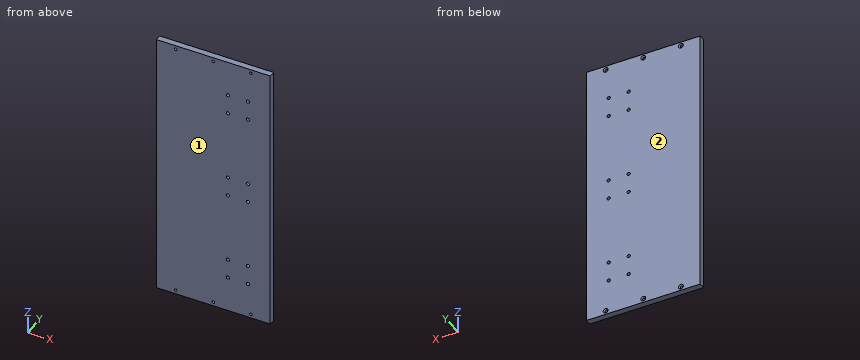
from build123d import *

# Parameters (mm, degrees)
SKETCH1_W                                    = 148
SKETCH1_H                                    = 344
BOSS_EXTRUDE1_DEPTH                          = 8
CSK_FOR_M3_COUNTERSUNK_FLAT_HEAD1_AT_2_COUNT = 2
CSK_FOR_M3_COUNTERSUNK_FLAT_HEAD1_AT_2_PITCH = 49
CSK_FOR_M3_COUNTERSUNK_FLAT_HEAD1_AT_3_COUNT = 2
CSK_FOR_M3_COUNTERSUNK_FLAT_HEAD1_AT_3_PITCH = 98
M5X0_8_TAPPED_HOLE1_D                        = 4.2
LPATTERN1_COUNT                              = 2
LPATTERN1_PITCH                              = 114
LPATTERN1_COL_COUNT                          = 2
LPATTERN1_COL_PITCH                          = 114


with BuildPart() as part:
    # Sketch1 → Boss-Extrude1 (new body)
    with BuildSketch(Plane(origin=(0, 0, 0), x_dir=(1, 0, 0), z_dir=(0, 1, 0))):
        Rectangle(SKETCH1_W, SKETCH1_H)
    extrude(amount=BOSS_EXTRUDE1_DEPTH)

    # Sketch3 → CSK for M3 Countersunk Flat Head1 (revolve, cut)
    with BuildSketch(Plane(origin=(-49, 8, 167), x_dir=(0, 0, 1), z_dir=(1, 0, 0))):
        Polygon((0, 0), (0, 16.021463052), (1.7, 15), (1.7, 1.45), (3.15, 0), align=None)
    csk_for_m3_countersunk_flat_head1 = revolve(axis=Axis((-49, 14.35, 167), (0, -1, 0)), mode=Mode.SUBTRACT)

    # CSK for M3 Countersunk Flat Head1 at 2: CSK for M3 Countersunk Flat Head1 ×2
    with Locations(*[(i * CSK_FOR_M3_COUNTERSUNK_FLAT_HEAD1_AT_2_PITCH, 0, 0) for i in range(1, CSK_FOR_M3_COUNTERSUNK_FLAT_HEAD1_AT_2_COUNT)]):
        add(csk_for_m3_countersunk_flat_head1, mode=Mode.SUBTRACT)

    # CSK for M3 Countersunk Flat Head1 at 3: CSK for M3 Countersunk Flat Head1 ×2
    with Locations(*[(i * CSK_FOR_M3_COUNTERSUNK_FLAT_HEAD1_AT_3_PITCH, 0, 0) for i in range(1, CSK_FOR_M3_COUNTERSUNK_FLAT_HEAD1_AT_3_COUNT)]):
        add(csk_for_m3_countersunk_flat_head1, mode=Mode.SUBTRACT)

    # Mirror1: CSK for M3 Countersunk Flat Head1 across plane
    add(csk_for_m3_countersunk_flat_head1.mirror(Plane.XY), mode=Mode.SUBTRACT)

    # Mirror1 copy 1 sketch → Mirror1 copy 1 (revolve, cut)
    with BuildSketch(Plane(origin=(0, 8, -167), x_dir=(0, 0, -1), z_dir=(1, 0, 0))):
        Polygon((0, 0), (0, -16.021463052), (1.7, -15), (1.7, -1.45), (3.15, 0), align=None)
    revolve(axis=Axis((0, 14.35, -167), (0, 1, 0)), mode=Mode.SUBTRACT)

    # Mirror1 copy 2 sketch → Mirror1 copy 2 (revolve, cut)
    with BuildSketch(Plane(origin=(49, 8, -167), x_dir=(0, 0, -1), z_dir=(1, 0, 0))):
        Polygon((0, 0), (0, -16.021463052), (1.7, -15), (1.7, -1.45), (3.15, 0), align=None)
    revolve(axis=Axis((49, 14.35, -167), (0, 1, 0)), mode=Mode.SUBTRACT)

    # M5x0.8 Tapped Hole1 (through all)
    with Locations(Plane(origin=(45, 8, -12.5), x_dir=(0, 0, 1), z_dir=(0, 1, 0))):
        with Locations((0, 0), (0, -26), (25, -26), (25, 0)):
            m5x0_8_tapped_hole1 = Hole(M5X0_8_TAPPED_HOLE1_D / 2)

    # LPattern1: M5x0.8 Tapped Hole1 ×2
    with Locations(*[(0, 0, i * LPATTERN1_PITCH) for i in range(1, LPATTERN1_COUNT)]):
        add(m5x0_8_tapped_hole1, mode=Mode.SUBTRACT)

    # LPattern1 col: M5x0.8 Tapped Hole1 ×2
    with Locations(*[(0, 0, -i * LPATTERN1_COL_PITCH) for i in range(1, LPATTERN1_COL_COUNT)]):
        add(m5x0_8_tapped_hole1, mode=Mode.SUBTRACT)


solid = part.part
Design review of the part built by this model. Coordinates are the model's own, in mm. Face numbers are marked on the shaded views. Coordinates: 2 decimals unless noted, no trailing zeros. Use one line per item in the form item = value. Start each with the question number.
(1) The part is to be moulded in two halves that separate along Y. For the marked faces 1 and 2, say which applies: +Y half, -Y half, draft (parallel to the pull), parting line (faces both ways), or undercut.
(2) Insertion check: pin 1 (6.5 mm diameter, centred on x = 45, z = 12.5, fed in from -Y); pin 2 (4.5 mm diameter, centred on x = 0, z = 167, fed in from +Y); pin 3 (2.5 mm diameter, centred on x = 49, z = 167, fed in from -Y). Each pin has a flat end and moves straight along its axis. Give the tip position at first contact, or say it passes through.
(3) For probe 1 along Z at (x, y) = (-49, 3); probe 2 along X at (y, z) = (5.25, 126.5); probe 3 along X at (y, z) = (3.5, 167), list the stretches that pass through material, from the lowest coordinate up.
Answer block:
q1.face_1 = -Y half
q1.face_2 = +Y half
q2.pin_1 = 0
q2.pin_2 = 7.1
q2.pin_3 = through
q3.probe_1 = -172 to -168.7, -165.3 to 165.3, 168.7 to 172
q3.probe_2 = -74 to 16.9, 21.1 to 42.9, 47.1 to 74
q3.probe_3 = -74 to -50.7, -47.3 to -1.7, 1.7 to 47.3, 50.7 to 74
